For this review, take the finished solid that the model builds, in its own axes (mm). Coordinates: 2 decimals unless noted, no trailing zeros. Order: outer loops, then holes, each group sorted by start corner. A loop starts at its lowest first (then second) coordinate and runs counter-clockwise, first axis right, second up. Notation, with made-up numbers: (-18, -28.75) -> (-7, -28.75) arc R11 ccw to (-7, -20.75) -> close; hole circle Ø2 at (-34, 78.25). An arc over 180 degrees is marked (long way). Return JSON: item names as keys, results as strings. Group by question number.
Item 1: For line 1 along Y through (x, z) = (-0.25, 114.5); line 2 along Y through (x, z) = (-1.65, 143); line 3 along X through (y, z) = (-0.15, 43), list the stretches that pass through material, from the lowest coordinate up.
Item 2: Insertion check: pin 1 (1.5 mm diameter, centred on y = 1, z = 93.5, fed in from -X); pin 2 (2 mm diameter, centred on x = -2, z = 93.5, fed in from +Y); pin 3 (2 mm diameter, centred on x = -2.5, z = 100.5, fed in from -Y). Each pin has a flat end and moves straight along its axis. Give the tip position at first contact, or say it passes through.
Item 3: Take a section at A-A (z = 83). Write out the cut boundary in (x, y).
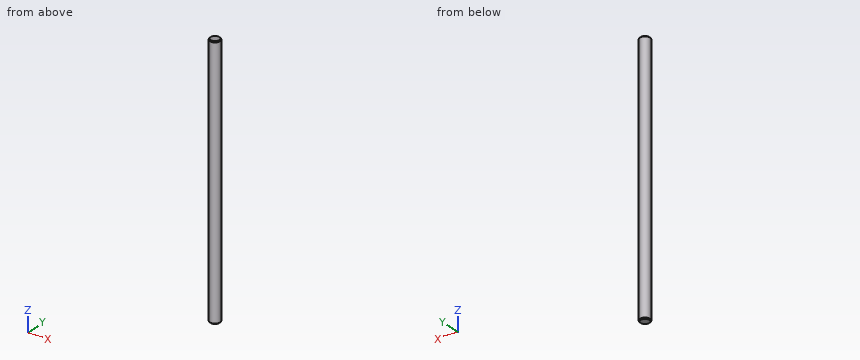
Autodesk Inventor part; units mm, degrees
ref_plane "YZ Plane" through (0, 0, 0) normal (1, 0, 0) x (0, 1, 0)
ref_plane "XZ Plane" through (0, 0, 0) normal (0, 1, 0) x (-1, 0, 0)
ref_plane "XY Plane" through (0, 0, 0) normal (0, 0, 1) x (1, 0, 0)
sketch "Sketch1" plane through (0, 0, 0) normal (0, 0, 1) x (1, 0, 0)
  circle A0 centre (0, 0) radius 3
  dimension "d0" = 6
extrude "Extrusion1" add sketch "Sketch1" along normal blind 150
chamfer "Chamfer1" distance 0.5 angle 45 1 edges at (-3, 0, 0)
chamfer "Chamfer2" distance 0.5 angle 45 1 edges at (-3, 0, 150)
properties part number "6mmx150mmSmoothRod"
Findings below:
{
 "1": {"line 1": "y = -2.99 to 2.99", "line 2": "y = -2.51 to 2.51", "line 3": "x = -3 to 3"},
 "2": {"pin 1": "stops at x = -2.99", "pin 2": "stops at y = 2.83", "pin 3": "stops at y = -2.6"},
 "3": {"outline": "circle Ø6 at (0, 0)"}
}
